Work out the finished part from the listing and answer in its coordinate system (mm). Face numbers are marked on the shaded views. A direction names the side the tool comes from. Coordinates: 2 decimals unless noted, no trailing zeros. Loops run counter-clockwise (first coordinate to the right, second up) from the corner with the lowest first, then second, coordinate; pieces in that order, holes last. Notation, with made-up numbers: (63, 18.25) - (78, 18.25) arc R18 cw to (78, 26.25) - close; hole circle Ø8 at (59.5, -1). An arc over 180 degrees is marked (long way). Write each question's results on one line, items separated by ' | '. Start each with the question number.
Item 1: Section C-C, the plane z = -8.5 is taken. Write down the section's boundary in (x, y).
Item 2: Section D-D, the plane y = 33 is taken. Write down the section's boundary in (x, z), plus the area to 3 significant figures.
Item 3: Each of these flat-tipped pins is pushed along its axis until it touches: pin 1 Ø6 at (x, y) = (-4.5, 8.5) entering from -Z; pin 2 Ø1.5 at (x, y) = (-9, 9) entering from +Z; pin 3 Ø5 at (y, z) = (28.5, 4.5) entering from -X; pin 4 Ø10 at (y, z) = (27.5, 8.5) entering from -X. Where does it stop, or does it pass through?
Item 4: A tool of negligible diameter and unlimited length cuts with its end or side. For the marked faces 1, 2 and 3, from which of +Z, -Z, +X, -X, +Y, -Y can it reach the whole face along a straight path? Write none if from no direction.
Item 5: Consider probe 1 along Y at (x, z) = (-3.75, 8.75); probe 2 along X at (y, z) = (43.75, 0); probe 3 along X at (y, z) = (33.5, 3.25). Determine where each line is inside the solid, lowest interval first. Write a range as [from, to].
Item 6: Section B-B, the plane x = -9 is taken. Write down the section's boundary in (y, z), plus the area to 3 significant figures.
Item 7: For a pull along Y with two mould halves and no side action, classify the marked faces 4, 5, 6 and 7 as +Y half, -Y half, draft (parallel to the pull), parting line (faces both ways), or undercut.
Item 8: Section A-A, the plane z = 0 is taken. Write down the section's boundary in (x, y), plus the area to 3 significant figures.
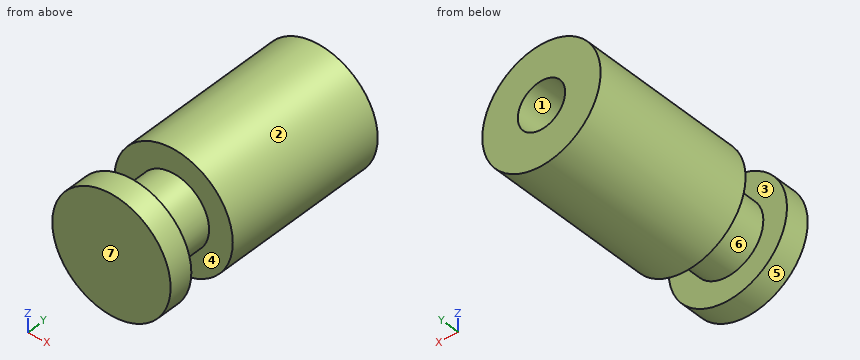
from build123d import *

# Parameters (mm, degrees)
SKETCH1_R           = 12.5
BOSS_EXTRUDE1_DEPTH = 50
SKETCH2_R           = 5
CUT_EXTRUDE1_DEPTH  = 20
SKETCH3_W           = 5
SKETCH3_H           = 10


with BuildPart() as part:
    # Sketch1 → Boss-Extrude1 (new body)
    with BuildSketch(Plane(origin=(0, 0, 0), x_dir=(1, 0, 0), z_dir=(0, 1, 0))):
        with Locations(Location((0, 0, 0), (0, 0, 270))):
            Circle(SKETCH1_R)
    extrude(amount=BOSS_EXTRUDE1_DEPTH)

    # Sketch2 → Cut-Extrude1 (cut)
    with BuildSketch(Plane(origin=(0, 50, 0), x_dir=(1, 0, 0), z_dir=(0, 1, 0))):
        with Locations(Location((0, 0, 0), (0, 0, 270))):
            Circle(SKETCH2_R)
    extrude(amount=-CUT_EXTRUDE1_DEPTH, mode=Mode.SUBTRACT)

    # Sketch3 → Cut-Revolve1 (revolve, cut)
    with BuildSketch(Plane(origin=(0, 0, 0), x_dir=(0, 0, -1), z_dir=(1, 0, 0)), mode=Mode.PRIVATE) as cut_revolve1_sk:
        with Locations((10, 10)):
            Rectangle(SKETCH3_W, SKETCH3_H)
    revolve(cut_revolve1_sk.sketch.rotate(Axis((0, 58.266357572, 0), (0, -1, 0)), 180), axis=Axis((0, 58.266357572, 0), (0, -1, 0)), mode=Mode.SUBTRACT)


solid = part.part
Answer key:
1) outline: (-9.17, 0) - (9.17, 0) - (9.17, 5) - (-9.17, 5) - close; (-9.17, 15) - (9.17, 15) - (9.17, 50) - (-9.17, 50) - close
2) outline: circle Ø25 at (0, 0); hole circle Ø10 at (0, 0) | area: 412 mm^2
3) pin 1: stops at z = -7.35 | pin 2: passes through | pin 3: stops at x = -12.34 | pin 4: stops at x = -12
4) face 1: +Y | face 2: +Y, -Y | face 3: none
5) probe 1: y = [0, 5], [15, 50] | probe 2: x = [-12.5, -5], [5, 12.5] | probe 3: x = [-12.07, -3.8], [3.8, 12.07]
6) outline: (0, -8.67) - (5, -8.67) - (5, 8.67) - (0, 8.67) - close; (15, -8.67) - (50, -8.67) - (50, 8.67) - (15, 8.67) - close | area: 694 mm^2
7) face 4: undercut | face 5: draft | face 6: undercut | face 7: -Y half
8) outline: (-12.5, 0) - (12.5, 0) - (12.5, 5) - (7.5, 5) - (7.5, 15) - (12.5, 15) - (12.5, 50) - (5, 50) - (5, 30) - (-5, 30) - (-5, 50) - (-12.5, 50) - (-12.5, 15) - (-7.5, 15) - (-7.5, 5) - (-12.5, 5) - close | area: 950 mm^2
